from build123d import *

# Parameters (mm, degrees)
F1_DEPTH = 15.7734
F2_R     = 10.16
F3_DEPTH = 15.7744
F4_DEPTH = 40.2336
F6_DEPTH = 40.2346
F7_R     = 3.302


with BuildPart() as f1:
    # F0 (on Front) → F1 (new body)
    with BuildSketch(Plane.XZ):
        with BuildLine():
            ThreePointArc((4.7064705882, 28.1847433836), (21.8061691049, 18.4667705344), (28.575, 0))
            ThreePointArc((28.575, 0), (21.8061691049, -18.4667705344), (4.7064705882, -28.1847433836))
            Line((4.7064705882, -28.1847433836), (57.2172352941, -19.4161565532))
            ThreePointArc((57.2172352941, -19.4161565532), (73.66, 0), (57.2172352941, 19.4161565532))
            Line((57.2172352941, 19.4161565532), (4.7064705882, 28.1847433836))
        make_face()
    extrude(amount=F1_DEPTH)

    # F2 (on face) → F3 (cut, through all)
    with BuildSketch(Plane.XZ.offset(15.7734)):
        with Locations((53.975, 0)):
            Circle(F2_R)
    extrude(amount=-F3_DEPTH, mode=Mode.SUBTRACT)

    # F0 (on Front) → F4 (join)
    with BuildSketch(Plane.XZ):
        with BuildLine():
            ThreePointArc((4.7064705882, -28.1847433836), (21.8061691049, -18.4667705344), (28.575, 0))
            ThreePointArc((28.575, 0), (21.8061691049, 18.4667705344), (4.7064705882, 28.1847433836))
            ThreePointArc((4.7064705882, 28.1847433836), (-28.575, 0), (4.7064705882, -28.1847433836))
        make_face()
    extrude(amount=F4_DEPTH)

    # F5 (on face) → F6 (cut, through all)
    with BuildSketch(Plane.XZ.offset(40.2336)):
        with BuildLine():
            ThreePointArc((13.4477648793, -4.826), (14.0760007986, -2.4492565746), (14.2875, 0))
            ThreePointArc((14.2875, 0), (14.0760007986, 2.4492565746), (13.4477648793, 4.826))
            Line((13.4477648793, 4.826), (-13.4477648793, 4.826))
            ThreePointArc((-13.4477648793, 4.826), (-14.2875, 0), (-13.4477648793, -4.826))
            Line((-13.4477648793, -4.826), (13.4477648793, -4.826))
        make_face()
        with BuildLine():
            Line((-13.4477648793, 4.826), (13.4477648793, 4.826))
            ThreePointArc((13.4477648793, 4.826), (0, 14.2875), (-13.4477648793, 4.826))
        make_face()
        with BuildLine():
            ThreePointArc((-13.4477648793, -4.826), (0, -14.2875), (13.4477648793, -4.826))
            Line((13.4477648793, -4.826), (-13.4477648793, -4.826))
        make_face()
        with BuildLine():
            ThreePointArc((13.4477648793, 4.826), (14.0760007986, 2.4492565746), (14.2875, 0))
            ThreePointArc((14.2875, 0), (14.0760007986, -2.4492565746), (13.4477648793, -4.826))
            Line((13.4477648793, -4.826), (18.5293, -4.826))
            Line((18.5293, -4.826), (18.5293, 4.826))
            Line((18.5293, 4.826), (13.4477648793, 4.826))
        make_face()
    extrude(amount=-F6_DEPTH, mode=Mode.SUBTRACT)

    # F7
    f7_edges = [f1.edges().sort_by_distance(p)[0] for p in [
        (-4.706471, -40.2336, 28.184743),
    ]]
    fillet(f7_edges, radius=F7_R)


solid = f1.part
Source: CAD feature listing. Evaluate the final solid. Frame: model axes, mm. A direction names the side the tool comes from. Give positions to 0.01 mm unless a question says otherwise; leave off trailing zeros. Write each loop counter-clockwise with the first axis right and the second up, starting at its lowest first coordinate (ties: lowest second). Pieces come first, ordered by that corner, then holes. Notation, with made-up numbers: M 12,69.5 L 54,69.5 A25 ccw 54,103.5 Z; hole C 71.5,67 d3. An arc over 180 degrees is marked long. Return JSON: item names as keys, results as strings. Group by question number.
1) Cut plane C-C, the plane x = 50. Output: boundary loops of the cut face in (y, z), plus the area to 3 significant figures.
2) Pull-direction query (Z, two-part tool) for faces 3 (the face through (11, -40.234, -11)), 4 (the face through (16, -20, 4.826)), 5 (the face through (73.656, -7.776, -0.387)), 6 (the face through (31.33, -7.78, 23.74)); classes: pulls with the +Z half, pulls with the -Z half, needs draft (parallel to the pull), parting line crosses it, or undercut.
3) Material intervals for line 1 along Y through (x, z) = (40.5, 4); line 2 along X through (y, z) = (-22.5, -12); line 3 along Z through (x, y) = (11.5, -32), sorted ascending. Write a range as [from, to].
4) Set-up query: faces 1 (the face through (18.529, -20, 0)), 2 (the face through (22, 0, 0)). Return all of +Z, -Z, +X, -X, +Y, -Y with unobstructed straight access to the full face (end or side cutting, diameter ignored); none if empty.
5) Pin query (flat end, axial travel): P1, Ø4, axis at y = -5, z = -13.5, coming from the +X side; P2, Ø1, axis at x = 29.5, y = -14.5, coming from the -Z side; P3, Ø1.5, axis at x = -12, y = -28, coming from the +Z side. Return the tip coordinate at first contact, or that it passes through.
6) Cut plane D-D, the plane z = -2.5. Give the number of separate pieces and of enclosed holes in the cut face, plus the area to 3 significant figures.
7) Cut plane B-B, the plane x = 63. Output: boundary loops of the cut face in (y, z), plus the area to 3 significant figures.
Recorded:
{
 "1": {"outline": "M -15.77,-20.62 L 0,-20.62 L 0,-9.35 L -15.77,-9.35 Z; M -15.77,9.35 L 0,9.35 L 0,20.62 L -15.77,20.62 Z", "area": "356 mm²"},
 "2": {"face 3": "needs draft", "face 4": "undercut", "face 5": "parting line crosses it", "face 6": "pulls with the +Z half"},
 "3": {"line 1": "y = [-15.77, 0]", "line 2": "x = [-25.93, -7.75], [7.75, 25.93]", "line 3": "z = [-26.16, -8.48], [8.48, 26.16]"},
 "4": {"face 1": "+Y, -Y", "face 2": "+Z, -Z, +X, -X, +Y"},
 "5": {"P1": "stops at x = 69.95", "P2": "stops at z = -24.13", "P3": "stops at z = 26.27"},
 "6": {"separate pieces": "3", "enclosed holes": "0", "area": "1,370 mm²"},
 "7": {"outline": "M -15.77,-17.49 L 0,-17.49 L 0,-4.67 L -15.77,-4.67 Z; M -15.77,4.67 L 0,4.67 L 0,17.49 L -15.77,17.49 Z", "area": "405 mm²"}
}
